from build123d import *

# Parameters (mm, degrees)
PAD001_DEPTH      = 129.237
PAD001_DEPTH_BACK = 129.237
SKETCH005_R       = 3.175
POCKET002_DEPTH   = 1.6002
SKETCH010_R       = 3.175
POCKET003_DEPTH   = 1.6002


with BuildPart() as pocket003:
    # Sketch003 → Pad001 (new body, two sides)
    with BuildSketch(Plane(origin=(-129.237, 0, -38.1), x_dir=(1, 0, 0), z_dir=(0, 1, 0))) as pad001_sk:
        Polygon((0, 0), (38.1, 0), (38.1, -1.6002), (1.6002, -1.6002), (1.6002, -38.1), (0, -38.1), align=None)
    extrude(amount=PAD001_DEPTH)
    extrude(pad001_sk.sketch, amount=-PAD001_DEPTH_BACK)

    # Sketch005 → Pocket002 (cut)
    with BuildSketch(Plane(origin=(-129.237, 0, -38.1), x_dir=(0, 0, 1), z_dir=(-1, 0, 0))):
        with Locations((25.4, 105.4372)):
            Circle(SKETCH005_R)
        with Locations((14.3002, 116.537)):
            Circle(SKETCH005_R)
        with Locations((25.4, -105.4372)):
            Circle(SKETCH005_R)
        with Locations((14.3002, -116.537)):
            Circle(SKETCH005_R)
    extrude(amount=-POCKET002_DEPTH, mode=Mode.SUBTRACT)

    # Sketch010 → Pocket003 (cut)
    with BuildSketch(Plane(origin=(-129.237, 0, -38.1), x_dir=(-1, 0, 0), z_dir=(0, 0, -1))):
        with Locations((-23.7998, -65.0766)):
            Circle(SKETCH010_R)
        with Locations((-12.7, -76.2272)):
            Circle(SKETCH010_R)
        with Locations((-23.7998, 65.0766)):
            Circle(SKETCH010_R)
        with Locations((-12.7, 76.2272)):
            Circle(SKETCH010_R)
    extrude(amount=-POCKET003_DEPTH, mode=Mode.SUBTRACT)


with BuildPart() as part_mirroring:
    # Part__Mirroring: instance of Pocket003
    add(pocket003.part.mirror(Plane(origin=(0, 0, 0), x_dir=(0, -1, 0), z_dir=(1, 0, 0))))


with BuildPart() as part_mirroring_1:
    # Part__Mirroring placement: moved
    add(part_mirroring.part.moved(Location((0, 0.0127, 0))))


solid = part_mirroring_1.part
For this review, take the finished solid that the model builds, in its own axes (mm). A direction names the side the tool comes from. Round coordinates to 2 decimals unless told otherwise and drop trailing zeros. Loops run counter-clockwise (first coordinate to the right, second up) from the corner with the lowest first, then second, coordinate; pieces in that order, holes last. Notation, with made-up numbers: (43.25, 75.25) - (54.25, 75.25) arc R20 cw to (54.25, 96.25) - close; hole circle Ø2 at (-35.5, 4.25). An arc over 180 degrees is marked (long way). Put each result on its own line as item: value. Start each with the question number.
1. For faces 4 (the cylindrical face through (128.45, 102.35, -13.39)), 5 (the flat face through (127.637, 2, -19)), list the 3-axis set-ups (+Z, -Z, +X, -X, +Y, -Y) from which the entire face can be reached by the end or side of a thin tool; tool diameter is ignored.
2. Consider section B-B on y = -24.5. State the section outline as (x, z) points, plus the area to 3 significant figures.
3. Insertion check: P1, Ø12, axis at x = 114.5, y = -48.5, coming from the +Z side; P2, Ø10, axis at y = -116.52, z = -23.8, coming from the -X side. Each pin has a flat end and moves straight along its axis. Give the tip position at first contact, or say it passes through.
4. Consider section A-A on z = -12.7. State the section outline as (x, y) points, plus the area to 3 significant figures.
5. For probe 1 along Y at (x, z) = (128.9, -12.7); probe 2 along X at (y, z) = (-95, -15); probe 3 along Z at (x, y) = (125, 41), list the stretches that pass through material, from the lowest coordinate up. Write a range as [from, to].
6. Mouldability with a two-part tool opening along Z and no side actions: class faces 1 (the flat face through (109, 2, -36.5)), 2 (the flat face through (119, -129.224, -37)), 3 (the cylindrical face through (128.448, -113.376, -24.213)) as +Z half, -Z half, draft (parallel to the pull), parting line (faces both ways), or undercut.
Result sheet:
1. face 4: +X, -X
1. face 5: +Z, -X, +Y, -Y
2. outline: (91.14, -38.1) - (129.24, -38.1) - (129.24, 0) - (127.64, 0) - (127.64, -36.5) - (91.14, -36.5) - close
2. area: 119 mm^2
3. P1: z = -36.5
3. P2: x = 127.64
4. outline: (127.64, -129.22) - (129.24, -129.22) - (129.24, -108.6) - (127.64, -108.6) - close; (127.64, -102.25) - (129.24, -102.25) - (129.24, 102.27) - (127.64, 102.27) - close; (127.64, 108.62) - (129.24, 108.62) - (129.24, 129.25) - (127.64, 129.25) - close
4. area: 393 mm^2
5. probe 1: [-129.22, -108.6], [-102.25, 102.27], [108.62, 129.25]
5. probe 2: [127.64, 129.24]
5. probe 3: [-38.1, -36.5]
6. face 1: +Z half
6. face 2: draft
6. face 3: undercut
